Design review of the part built by this model. Coordinates are the model's own, in mm. A direction names the side the tool comes from. Coordinates: 2 decimals unless noted, no trailing zeros. Order: outer loops, then holes, each group sorted by start corner. A loop starts at its lowest first (then second) coordinate and runs counter-clockwise, first axis right, second up. Notation, with made-up numbers: (12.5, 35) - (52.5, 35) arc R30 ccw to (52.5, 57) - close; hole circle Ø2 at (-33.5, -17.75). An arc over 180 degrees is marked (long way). Write each question's results on one line, items separated by ' | '. Start each with the question number.
```python
from build123d import *

# Parameters (mm, degrees)
SKETCH1_W          = 9.652
SKETCH1_H          = 40.4622
EXTRUDE1_DEPTH     = 12.7
FILLET1_R          = 0.127
CUT_EXTRUDE1_DEPTH = 10.652
SKETCH5_R          = 1.7272
CUT_EXTRUDE2_DEPTH = 13.7


with BuildPart() as part:
    # Sketch1 → Extrude1 (new body)
    with BuildSketch(Plane(origin=(0, 0, 0), x_dir=(1, 0, 0), z_dir=(0, 1, 0))):
        with Locations((4.826, -20.2311)):
            Rectangle(SKETCH1_W, SKETCH1_H)
    extrude(amount=EXTRUDE1_DEPTH)

    # Sketch3 → Cut-Revolve1 (revolve, cut)
    with BuildSketch(Plane(origin=(4.826, 0, 0), x_dir=(0, 0, -1), z_dir=(1, 0, 0))):
        Polygon((-11.8872, 12.7), (-11.8872, 8.5344), (-10.2108, 8.5344), (-10.2108, 6.6548), (-10.629274995, 6.6548), (-11.0363, 0), (-7.9248, 0), (-7.9248, 12.7), align=None)
    revolve(axis=Axis((4.826, 31.679444444, 7.9248), (0, -1, 0)), mode=Mode.SUBTRACT)

    # Fillet1
    fillet1_edges = [part.edges().sort_by_distance(p)[0] for p in [
        (4.826, 6.6548, 5.220325005),
    ]]
    fillet(fillet1_edges, radius=FILLET1_R)

    # Sketch4 → Cut-Extrude1 (cut, through all)
    with BuildSketch(Plane(origin=(9.652, 0, 0), x_dir=(0, 0, -1), z_dir=(1, 0, 0))):
        Polygon((-40.4622, 5.08), (-40.4622, 12.7), (-15.8496, 12.7), align=None)
    extrude(amount=-CUT_EXTRUDE1_DEPTH, mode=Mode.SUBTRACT)

    # Sketch5 → Cut-Extrude2 (cut, through all)
    with BuildSketch(Plane.XZ):
        with Locations(Location((4.826, 36.4998, 0), (0, 0, 270))):  # turned: the seam where the file's is
            Circle(SKETCH5_R)
    extrude(amount=-CUT_EXTRUDE2_DEPTH, mode=Mode.SUBTRACT)


solid = part.part
```
(1) Tool access review of faces 5 (the face through (5.34, 3.37, 34.85)), 6 (the face through (7, 8.534, 10)): name each direction out of +Z, -Z, +X, -X, +Y, -Y from which nothing blocks a thin tool from reaching the whole face with its end or side.
(2) To check wall thickness, follow line 1 along Z through (x, y) = (5, 1); line 2 along Y through (x, z) = (6.25, 10); line 3 along X through (y, z) = (8.5, 9). State the ranges of each line that lie inside material, in increasing order. Write a range as [from, to].
(3) Mouldability with a two-part tool opening along X and no side actions: class faces 1 (the face through (9.652, 5, 16)), 2 (the face through (5, 0, 20)), 3 (the face through (5.702, 7.581, 10.036)), 4 (the face through (6.344, 10.588, 11.585)) as +X half, -X half, draft (parallel to the pull), parting line (faces both ways), or undercut.
(4) Take a section at D-D (z = 17). State the section outline as (x, y) points, plus the area to 3 significant figures.
(5) Take a section at B-B (y = 4.5). State the section outline as (x, z) points, plus the area to 3 significant figures.
(6) Take a section at C-C (z = 29). State the section outline as (x, y) points, plus the area to 3 significant figures.
(7) Clearance check with flat-ended pins moving along their axes: pin 1 (1.5 mm diameter, centred on y = 9.5, z = 33, fed in from -X); pin 2 (2.5 mm diameter, centred on x = 4, z = 9, fed in from +Y). State where each tip first meets the part, or that it passes through.
(8) Take a section at A-A (y = 9.5). State the section outline as (x, z) points, plus the area to 3 significant figures.
Worked out:
1) face 5: +Y, -Y | face 6: +Y
2) line 1: [0, 4.88], [10.97, 34.78], [38.22, 40.46] | line 2: [6.65, 8.53] | line 3: [0, 2.81], [6.84, 9.65]
3) face 1: +X half | face 2: draft | face 3: undercut | face 4: undercut
4) outline: (0, 0) - (9.65, 0) - (9.65, 12.34) - (0, 12.34) - close | area: 119 mm^2
5) outline: (0, 0) - (9.65, 0) - (9.65, 40.46) - (0, 40.46) - close; hole circle Ø5.67 at (4.83, 7.92); hole circle Ø3.45 at (4.83, 36.5) | area: 356 mm^2
6) outline: (0, 0) - (9.65, 0) - (9.65, 8.63) - (0, 8.63) - close | area: 83.3 mm^2
7) pin 1: through | pin 2: y = 8.53
8) outline: (0, 0) - (9.65, 0) - (9.65, 26.19) - (0, 26.19) - close; hole circle Ø7.92 at (4.83, 7.92) | area: 203 mm^2
